Read the model definition and answer for the solid it produces. Units are mm, in the model's axes. Face numbers are marked on the shaded views. A direction names the side the tool comes from. Coordinates: 2 decimals unless noted, no trailing zeros. Write each loop counter-clockwise with the first axis right and the second up, starting at its lowest first coordinate (ties: lowest second). Pieces come first, ordered by that corner, then holes. Notation, with made-up numbers: (27.25, 6) - (74.25, 6) arc R30 ccw to (74.25, 41) - close; hole circle Ø7 at (24.25, -6.75). An arc over 180 degrees is marked (long way). Use a Markdown table: item, result.
from build123d import *

# Parameters (mm, degrees)
ESQUISSE1_W                                 = 5
ESQUISSE1_H                                 = 20
BOSS_EXTRU_1_DEPTH                          = 80
BOSS_EXTRU_1_2_DEPTH                        = 80
ESQUISSE1_3_W                               = 61.5
ESQUISSE1_3_H                               = 20
BOSS_EXTRU_2_DEPTH                          = 8
ESQUISSE3_R                                 = 2.75
ENL_V_MAT_EXTRU_2_DEPTH                     = 85
ESQUISSE4_R                                 = 2.6
ESQUISSE4_R_2                               = 1.8
ENL_V_MAT_EXTRU_3_DEPTH                     = 10
CONG_4_R                                    = 10
ESQUISSE6_R                                 = 1.6
TROUS_PALONNIER_GRABCAD_M3_ENTRAXE_14_DEPTH = 103.870063673
NERVURE2_REACH                              = 103.401
ESQUISSE9_WALL_W                            = 40
ESQUISSE9_WALL_H                            = 10
ESQUISSE10_R                                = 3.5
ENL_V_MAT_EXTRU_4_DEPTH                     = 2
ENL_V_START                                 = -2
ESQUISSE11_R                                = 3.5
ENL_V_MAT_EXTRU_5_DEPTH                     = 2


with BuildPart() as part:
    # Esquisse1 → Boss.-Extru.1 (new body)
    with BuildSketch(Plane.XY):
        with Locations((2.5, 10)):
            Rectangle(ESQUISSE1_W, ESQUISSE1_H)
    extrude(amount=BOSS_EXTRU_1_DEPTH)



with BuildPart() as body_2:
    # Esquisse1 → Boss.-Extru.1 2 (new body)
    with BuildSketch(Plane.XY):
        with Locations((59, 10)):
            Rectangle(ESQUISSE1_W, ESQUISSE1_H)
    extrude(amount=BOSS_EXTRU_1_2_DEPTH)


with BuildPart() as part_1:
    add(part.part)

    add(body_2.part)  # Boss.-Extru.2 merges body 2
    # Esquisse1<3> → Boss.-Extru.2 (add)
    with BuildSketch(Plane.XY):
        with Locations((30.75, 10)):
            Rectangle(ESQUISSE1_3_W, ESQUISSE1_3_H)
    extrude(amount=-BOSS_EXTRU_2_DEPTH)

    # Esquisse3 → Enlèv. mat.-Extru.2 (cut)
    with BuildSketch(Plane(origin=(61.5, 0, 0), x_dir=(0, 0, -1), z_dir=(1, 0, 0))):
        with Locations((-68.927874881, 10)):
            Circle(ESQUISSE3_R)
    extrude(amount=-ENL_V_MAT_EXTRU_2_DEPTH, mode=Mode.SUBTRACT)

    # Esquisse4 → Enlèv. mat.-Extru.3 (cut)
    with BuildSketch(Plane(origin=(0, 0, -8), x_dir=(-1, 0, 0), z_dir=(0, 0, -1))):
        with Locations((-30.75, 10)):
            Circle(ESQUISSE4_R)
        with Locations((-37.75, 10)):
            Circle(ESQUISSE4_R_2)
        with Locations((-23.75, 10)):
            Circle(ESQUISSE4_R_2)
    extrude(amount=-ENL_V_MAT_EXTRU_3_DEPTH, mode=Mode.SUBTRACT)

    # Congé4
    cong_4_edges = [part_1.edges().sort_by_distance(p)[0] for p in [
        (2.5, 20, 80),
        (2.5, 0, 80),
        (59, 0, 80),
        (59, 20, 80),
    ]]
    fillet(cong_4_edges, radius=CONG_4_R - 0.0001)  # a hair under: the kernel refuses the full size

    # Esquisse6 → Trous palonnier GrabCAD M3 entraxe 14 (cut, through all)
    with BuildSketch(Plane(origin=(0, 0, 0), x_dir=(0, 0, -1), z_dir=(1, 0, 0))):
        with Locations((-75.927874881, 10)):
            Circle(ESQUISSE6_R)
        with Locations((-68.927874881, 17)):
            Circle(ESQUISSE6_R)
        with Locations((-61.927874881, 10)):
            Circle(ESQUISSE6_R)
        with Locations((-68.927874881, 3)):
            Circle(ESQUISSE6_R)
    extrude(amount=TROUS_PALONNIER_GRABCAD_M3_ENTRAXE_14_DEPTH, mode=Mode.SUBTRACT)

    # Esquisse9 wall → Nervure2 (add, up to next)
    with BuildSketch(Plane(origin=(49.659597134, 10, 18.793852416), x_dir=(0.342020143329, 0, 0.939692620785), z_dir=(-0.939692620785, 0, 0.342020143329)), mode=Mode.PRIVATE) as nervure2_sk1:
        Rectangle(ESQUISSE9_WALL_W, ESQUISSE9_WALL_H)
    nervure2_tool1 = extrude(nervure2_sk1.sketch, amount=-NERVURE2_REACH, mode=Mode.PRIVATE) - part_1.part
    nervure2 = nervure2_tool1.solids().sort_by_distance((49.659597134, 10, 18.793852416))[0]
    add(nervure2)

    # Symétrie1: Nervure2 across plane
    add(nervure2.mirror(Plane.ZY.offset(-30)))

    # Esquisse10 → Enlèv. mat.-Extru.4 (cut)
    with BuildSketch(Plane(origin=(61.5, 0, 0), x_dir=(0, 0, -1), z_dir=(1, 0, 0))):
        with Locations((-68.927874881, 10)):
            Circle(ESQUISSE10_R)
    extrude(amount=-ENL_V_MAT_EXTRU_4_DEPTH, mode=Mode.SUBTRACT)

    # Esquisse11 → Enlèv. mat.-Extru.5 (cut)
    with BuildSketch(Plane.ZY.offset(ENL_V_START)):
        with Locations(Location((68.927874881, 10, 0), (0, 0, 180))):
            Circle(ESQUISSE11_R)
    extrude(amount=ENL_V_MAT_EXTRU_5_DEPTH, mode=Mode.SUBTRACT)


solid = part_1.part
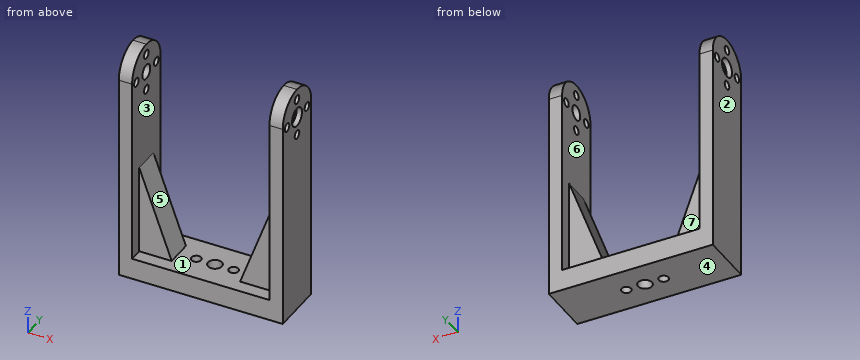
(1) A cutting plane is placed at C-C, the plane x = 23.75. Write down the section's boundary in (y, z), and give its area (3 significant figures).
Report:
| item | result |
|---|---|
| outline | (0, -8) - (8.2, -8) - (8.2, 0) - (0, 0) - close; (11.8, -8) - (20, -8) - (20, 0) - (11.8, 0) - close |
| area | 131 mm² |
(2) A cutting plane is placed at A-A, the plane x = 30.75. Write down the section's boundary in (y, z).
Report:
| item | result |
|---|---|
| outline | (0, -8) - (7.4, -8) - (7.4, 0) - (0, 0) - close; (12.6, -8) - (20, -8) - (20, 0) - (12.6, 0) - close |
(3) Straight lines are drawn through the part: L1, parallel to Y at x = 30.75, z = -5.5; L2, parallel to X at y = 2.25, z = 28.5; L3, parallel to Z at x = 38, y = 12.5. For each, find the intervals that lie inside material, in ascending order.
Report:
| item | result |
|---|---|
| L1 | y = 0 to 7.4, 12.6 to 20 |
| L2 | x = 0 to 5, 56.5 to 61.5 |
| L3 | z = -8 to 0 |
(4) For the marked faces 5, 6 and 7, determine the directions among +Z, -Z, +X, -X, +Y, -Y from which every point of the face is accessible in a straight line to the end or side of a thin tool.
Report:
| item | result |
|---|---|
| face 5 | +Z, +Y, -Y |
| face 6 | +Z |
| face 7 | +Z, +Y |
(5) The mould has two halves that part along X. Classify the marked faces 1, 2, 3 and 4: pulls with the +X half, pulls with the -X half, needs draft (parallel to the pull), parting line crosses it, or undercut.
Report:
| item | result |
|---|---|
| face 1 | undercut |
| face 2 | pulls with the -X half |
| face 3 | undercut |
| face 4 | needs draft |
(6) A cutting plane is placed at D-D, the plane x = 44. Write down the section's boundary in (y, z), and give its area (3 significant figures).
Report:
| item | result |
|---|---|
| outline | (0, -8) - (20, -8) - (20, 0) - (15, 0) - (15, 3.24) - (5, 3.24) - (5, 0) - (0, 0) - close |
| area | 192 mm² |
(7) Each of these flat-tipped pins is pushed along its axis until it touches: P1, Ø1.5, axis at y = 5.5, z = 46.5, coming from the -X side; P2, Ø1, axis at x = 29, y = 3.5, coming from the +Z side; P3, Ø15, axis at x = 48.5, z = 12, coming from the +Y side; P4, Ø1.9, axis at y = 17, z = 68.93, coming from the -X side. Where does it stop, or does it pass through?
Report:
| item | result |
|---|---|
| P1 | stops at x = 0 |
| P2 | stops at z = 0 |
| P3 | stops at y = 15 |
| P4 | passes through |
(8) A cutting plane is placed at B-B, the plane y = 17. Write down the section's boundary in (x, z), and give its area (3 significant figures).
Report:
| item | result |
|---|---|
| outline | (0, -8) - (61.5, -8) - (61.5, 67.33) - (56.5, 67.33) - (56.5, 0) - (5, 0) - (5, 67.33) - (0, 67.33) - close; (0, 70.53) - (5, 70.53) - (5, 77.14) - (0, 77.14) - close; (56.5, 70.53) - (61.5, 70.53) - (61.5, 77.14) - (56.5, 77.14) - close |
| area | 1,230 mm² |
